The listing builds one solid part. Answer for the finished solid, in the listing's coordinates (mm). Face numbers are marked on the shaded views. A direction names the side the tool comes from. Give positions to 0.01 mm unless a question says otherwise; leave off trailing zeros. Loops run counter-clockwise (first coordinate to the right, second up) from the corner with the lowest first, then second, coordinate; pieces in that order, holes last. Notation, with made-up numbers: M 49,36.5 L 94,36.5 A21 cw 94,41.5 Z; hole C 28,82 d2. An arc over 180 degrees is marked long. One line per item, written item: value. Start each with the question number.
Q1. The mould has two halves that part along Z. Classify the marked faces 4, 5 and 6: +Z half, -Z half, draft (parallel to the pull), parting line (faces both ways), or undercut.
Q2. Flat-ended cylindrical pins translate along their axes: pin 1 (1.6 mm diameter, centred on y = 3.5, z = 2.5, fed in from +X); pin 2 (1 mm diameter, centred on x = -1, z = 0.5, fed in from +Y); pin 3 (1.6 mm diameter, centred on y = 4.5, z = 2, fed in from -X). Find the tip coordinate at first contact, or state that the pin passes through.
Q3. A cutting plane is placed at A-A, the plane z = 2.35. Determine the outline of the cut face in (x, y), and give its area (3 significant figures).
Q4. For the marked faces 1, 2 and 3, determine the directions among +Z, -Z, +X, -X, +Y, -Y from which every point of the face is accessible in a straight line to the end or side of a thin tool.
Q5. Consider L1, parallel to Z at x = 1.3, y = 4.25; L2, parallel to Y at x = 0.85, z = 1.8; L3, parallel to X at y = 3.5, z = 2.85. Determine where each line is inside the solid, lowest interval first.
from build123d import *

# Parameters (mm, degrees)
F1_DEPTH = 1
F2_W     = 0.9661824606
F2_H     = 2.1
F3_DEPTH = 2
F4_W     = 0.85
F4_H     = 4.2
F5_DEPTH = 0.5
F6_SIZE  = 0.25


with BuildPart() as f1:
    # F0 (on Top) → F1 (new body)
    with BuildSketch(Plane.XY):
        with BuildLine():
            Line((0, 5.7256516985), (-2, 5.7256516985))
            add(Edge.make_bspline(
                [(-2, 5.7256516985), (-2.0680379738, 4.3142188256), (-1.4793331486, 2.1693367722), (-1, 1.0774956806)],
                knots=[0.49395691, 0.49395691, 0.49395691, 0.49395691, 0.8191677941, 0.8191677941, 0.8191677941, 0.8191677941], degree=3))
            Line((-1, 1.0774956806), (0, 1.0774956806))
            Line((0, 1.0774956806), (0, 5.7256516985))
        make_face()
        with BuildLine():
            Line((0, 8.7250128189), (-0.45, 8.7250128189))
            add(Edge.make_bspline(
                [(-0.45, 8.7250128189), (-0.6863850918, 8.530402377), (-1.3369422342, 7.7719026331), (-1.9532092441, 6.6963156863), (-2, 5.7256516985)],
                knots=[0.1083102347, 0.1083102347, 0.1083102347, 0.1083102347, 0.2703044079, 0.49395691, 0.49395691, 0.49395691, 0.49395691], degree=3))
            Line((-2, 5.7256516985), (0, 5.7256516985))
            Line((0, 5.7256516985), (0, 8.7250128189))
        make_face()
        with BuildLine():
            Line((0.45, 8.7250128189), (0, 8.7250128189))
            Line((0, 8.7250128189), (0, 5.7256516985))
            Line((0, 5.7256516985), (2, 5.7256516985))
            add(Edge.make_bspline(
                [(0.45, 8.7250128189), (0.6863850918, 8.530402377), (1.3369422342, 7.7719026331), (1.9532092441, 6.6963156863), (2, 5.7256516985)],
                knots=[0.1083102347, 0.1083102347, 0.1083102347, 0.1083102347, 0.2703044079, 0.49395691, 0.49395691, 0.49395691, 0.49395691], degree=3))
        make_face()
        with BuildLine():
            Line((2, 5.7256516985), (0, 5.7256516985))
            Line((0, 5.7256516985), (0, 1.0774956806))
            Line((0, 1.0774956806), (1, 1.0774956806))
            add(Edge.make_bspline(
                [(2, 5.7256516985), (2.0680379738, 4.3142188256), (1.4793331486, 2.1693367722), (1, 1.0774956806)],
                knots=[0.49395691, 0.49395691, 0.49395691, 0.49395691, 0.8191677941, 0.8191677941, 0.8191677941, 0.8191677941], degree=3))
        make_face()
        with BuildLine():
            Line((1, 1.0774956806), (0, 1.0774956806))
            Line((0, 1.0774956806), (0, 0))
            add(Edge.make_bspline(
                [(1, 1.0774956806), (0.7334687279, 0.4703818268), (0.5007537712, 0.188854692), (0, 0)],
                knots=[0.8191677941, 0.8191677941, 0.8191677941, 0.8191677941, 1, 1, 1, 1], degree=3))
        make_face()
        with BuildLine():
            Line((0, 1.0774956806), (-1, 1.0774956806))
            add(Edge.make_bspline(
                [(-1, 1.0774956806), (-0.7334687279, 0.4703818268), (-0.5007537712, 0.188854692), (0, 0)],
                knots=[0.8191677941, 0.8191677941, 0.8191677941, 0.8191677941, 1, 1, 1, 1], degree=3))
            Line((0, 0), (0, 1.0774956806))
        make_face()
        with BuildLine():
            add(Edge.make_bspline(
                [(0, 9), (0.150392861, 8.929814249), (0.2919515698, 8.8551304782), (0.45, 8.7250128189)],
                knots=[0, 0, 0, 0, 0.1083102347, 0.1083102347, 0.1083102347, 0.1083102347], degree=3))
            Line((0, 9), (0, 8.7250128189))
            Line((0, 8.7250128189), (0.45, 8.7250128189))
        make_face()
        with BuildLine():
            Line((0, 8.7250128189), (0, 9))
            add(Edge.make_bspline(
                [(0, 9), (-0.150392861, 8.929814249), (-0.2919515698, 8.8551304782), (-0.45, 8.7250128189)],
                knots=[0, 0, 0, 0, 0.1083102347, 0.1083102347, 0.1083102347, 0.1083102347], degree=3))
            Line((-0.45, 8.7250128189), (0, 8.7250128189))
        make_face()
    extrude(amount=F1_DEPTH)

    # F2 (on face) → F3 (join)
    with BuildSketch(Plane.XY.offset(1)):
        Polygon((-0.7338175394, 2.4), (0, 2.4), (0, 4.5), (0.9661824606, 4.5), (0.9661824606, 6.6), (-0.7338175394, 6.6), align=None)
        with Locations((0.4830912303, 3.45)):
            Rectangle(F2_W, F2_H)
    extrude(amount=F3_DEPTH)

    # F4 (on face) → F5 (join)
    with BuildSketch(Plane.XY.offset(3)):
        Polygon((0.1161824606, 6.6), (0.1161824606, 6.78964095), (-0.8687144145, 6.78964095), (-0.8687144145, 2.28964095), (0.1161824606, 2.28964095), (0.1161824606, 2.4), (-0.7338175394, 2.4), (-0.7338175394, 6.6), align=None)
        with Locations((-0.3088175394, 4.5)):
            Rectangle(F4_W, F4_H)
        with Locations((0.5411824606, 4.5)):
            Rectangle(F4_W, F4_H)
        Polygon((1.1312855855, 6.78964095), (0.1161824606, 6.78964095), (0.1161824606, 6.6), (0.9661824606, 6.6), (0.9661824606, 2.4), (0.1161824606, 2.4), (0.1161824606, 2.28964095), (1.1312855855, 2.28964095), align=None)
    extrude(amount=F5_DEPTH)

    # F6
    f6_edges = [f1.edges().sort_by_distance(p)[0] for p in [
        (0.131286, 2.289641, 3.5),
        (1.131286, 4.539641, 3.5),
        (0.131286, 6.789641, 3.5),
        (-0.868714, 4.539641, 3.5),
    ]]
    chamfer(f6_edges, length=F6_SIZE)


solid = f1.part
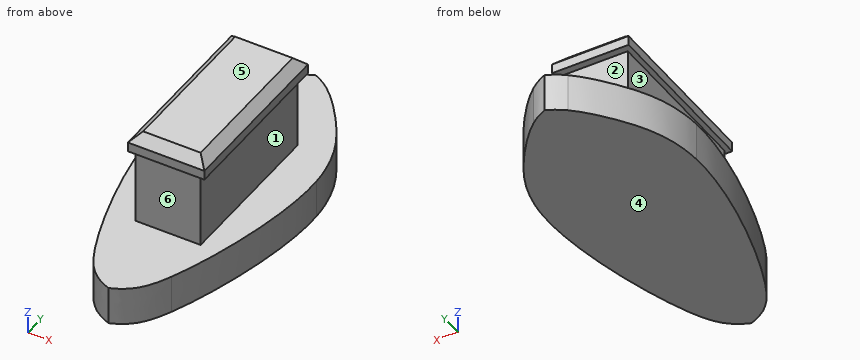
Answer block:
1. face 4: -Z half
1. face 5: +Z half
1. face 6: undercut
2. pin 1: x = 1.13
2. pin 2: y = 8.68
2. pin 3: x = -0.73
3. outline: M -0.73,2.4 L 0.97,2.4 L 0.97,6.6 L -0.73,6.6 Z
3. area: 7.14 mm^2
4. face 1: +X, +Y, -Y
4. face 2: +X, -X, +Y
4. face 3: -X, +Y, -Y
5. L1: 0 to 1
5. L2: 2.4 to 6.6
5. L3: -0.73 to 0.97
